Could you check a few things on this model? Use its own coordinates, in mm. Give positions to 0.01 mm unless a question says otherwise; leave off trailing zeros. Write each loop counter-clockwise with the first axis right and the second up, starting at its lowest first coordinate (ties: lowest second). Pieces come first, ordered by that corner, then holes. Notation, with made-up numbers: (-39, -20) - (-15, -20) arc R17 ccw to (-15, -16) - close; hole circle Ø1 at (-3, -3). An arc over 180 degrees is marked (long way). Use one line per item in the form item = value.
```python
from build123d import *

# Parameters (mm, degrees)
SKETCH_1_W          = 8
SKETCH_1_H          = 8
EXTRUDE_1_DEPTH     = 20
CUT_EXTRUDE_1_REACH = 23.909
SKETCH_2_R          = 1.5
CUT_EXTRUDE_2_REACH = 23.909
SKETCH_3_R          = 1.5


with BuildPart() as part:
    # 草图1 → 凸台-拉伸1 (new, symmetric)
    with BuildSketch(Plane.XY):
        Rectangle(SKETCH_1_W, SKETCH_1_H)
    extrude(amount=EXTRUDE_1_DEPTH, both=True)

    # 草图2 → 切除-拉伸1 (cut, up to next)
    with BuildSketch(Plane(origin=(4, 0, 0), x_dir=(0, 0, -1), z_dir=(1, 0, 0)), mode=Mode.PRIVATE) as cut_extrude_1_sk1:
        with Locations(Location((-15, 0, 0), (0, 0, 90))):
            Circle(SKETCH_2_R)
    cut_extrude_1_tool1 = extrude(cut_extrude_1_sk1.sketch, amount=-CUT_EXTRUDE_1_REACH, mode=Mode.PRIVATE) & part.part
    # 草图2 → 切除-拉伸1 (cut, up to next)
    with BuildSketch(Plane(origin=(4, 0, 0), x_dir=(0, 0, -1), z_dir=(1, 0, 0)), mode=Mode.PRIVATE) as cut_extrude_1_sk2:
        with Locations(Location((5, 0, 0), (0, 0, 90))):
            Circle(SKETCH_2_R)
    cut_extrude_1_tool2 = extrude(cut_extrude_1_sk2.sketch, amount=-CUT_EXTRUDE_1_REACH, mode=Mode.PRIVATE) & part.part
    add(cut_extrude_1_tool1.solids().sort_by_distance((4, 0, 15))[0], mode=Mode.SUBTRACT)
    add(cut_extrude_1_tool2.solids().sort_by_distance((4, 0, -5))[0], mode=Mode.SUBTRACT)

    # 草图3 → 切除-拉伸2 (cut, up to next)
    with BuildSketch(Plane(origin=(0, 4, 0), x_dir=(1, 0, 0), z_dir=(0, 1, 0)), mode=Mode.PRIVATE) as cut_extrude_2_sk1:
        with Locations(Location((0, 15, 0), (0, 0, 270))):
            Circle(SKETCH_3_R)
    cut_extrude_2_tool1 = extrude(cut_extrude_2_sk1.sketch, amount=-CUT_EXTRUDE_2_REACH, mode=Mode.PRIVATE) & part.part
    # 草图3 → 切除-拉伸2 (cut, up to next)
    with BuildSketch(Plane(origin=(0, 4, 0), x_dir=(1, 0, 0), z_dir=(0, 1, 0)), mode=Mode.PRIVATE) as cut_extrude_2_sk2:
        with Locations(Location((0, -5, 0), (0, 0, 270))):
            Circle(SKETCH_3_R)
    cut_extrude_2_tool2 = extrude(cut_extrude_2_sk2.sketch, amount=-CUT_EXTRUDE_2_REACH, mode=Mode.PRIVATE) & part.part
    add(cut_extrude_2_tool1.solids().sort_by_distance((0, 4, -15))[0], mode=Mode.SUBTRACT)
    add(cut_extrude_2_tool2.solids().sort_by_distance((0, 4, 5))[0], mode=Mode.SUBTRACT)


solid = part.part
```
1. Imagine slicing it at C-C, the plane x = 0.5. List the corners of the cut face in (y, z) for me, and give its area (3 significant figures).
Response values:
outline = (-4, -20) - (4, -20) - (4, -16.41) - (-4, -16.41) - close; (-4, -13.59) - (4, -13.59) - (4, 3.59) - (-4, 3.59) - close; (-4, 6.41) - (4, 6.41) - (4, 20) - (-4, 20) - close; hole circle Ø3 at (0, -5); hole circle Ø3 at (0, 15)
area = 261 mm²
2. If we mould it in two halves opening along X, with no side actions, what happens to faces 1 (the face through (-4, 0, 0)), 2 (the face through (0, 0, 20)), 3 (the face through (0.07, 0.06, -16.5))? For each: pulls with the +X half, pulls with the -X half, needs draft (parallel to the pull), parting line crosses it, or undercut.
Response values:
face_1 = pulls with the -X half
face_2 = needs draft
face_3 = undercut
3. Imagine slicing it at B-B, the plane z = -15. List the corners of the cut face in (x, y) for me.
Response values:
outline = (-4, -4) - (-1.5, -4) - (-1.5, 4) - (-4, 4) - close; (1.5, -4) - (4, -4) - (4, 4) - (1.5, 4) - close
4. Imagine slicing it at A-A, the plane y = 0. List the corners of the cut face in (x, z) for me, and give its area (3 significant figures).
Response values:
outline = (-4, -20) - (4, -20) - (4, -6.5) - (-4, -6.5) - close; (-4, -3.5) - (4, -3.5) - (4, 13.5) - (-4, 13.5) - close; (-4, 16.5) - (4, 16.5) - (4, 20) - (-4, 20) - close; hole circle Ø3 at (0, -15); hole circle Ø3 at (0, 5)
area = 258 mm²
5. If I drill on line 1 (Z direction, x = -3, y = -1); line 2 (Z direction, x = -1.25, y = -3); line 3 (X direction, y = 1.5, z = 5.5), over which ranges is the centre line in solid material (lowest first)? Write a range as from..to.
Response values:
line_1 = -20..-6.12, -3.88..13.88, 16.12..20
line_2 = -20..-15.83, -14.17..4.17, 5.83..20
line_3 = -4..-1.41, 1.41..4
6. Imagine slicing it at D-D, the plane x = -2. List the corners of the cut face in (y, z) for me.
Response values:
outline = (-4, -20) - (4, -20) - (4, 20) - (-4, 20) - close; hole circle Ø3 at (0, -5); hole circle Ø3 at (0, 15)
